from build123d import *

# Parameters (mm, degrees)
F2_R = 10


with BuildPart() as f1:
    # F0 (on Front) → F1 (revolve)
    with BuildSketch(Plane.XZ):
        with BuildLine():
            Line((-119.485281, 0), (-30, 0))
            Line((-30, 0), (-30, 75))
            ThreePointArc((-30, 75), (-33.703899, 80.543277), (-40.242641, 79.242641))
            Line((-40.242641, 79.242641), (-119.485281, 0))
        make_face()
    revolve(axis=Axis((0, 0, 64.130453), (0, 0, 1)))

    # F2 (on Front) → F3 (revolve, cut)
    with BuildSketch(Plane.XZ):
        with Locations((-70, 50)):
            Circle(F2_R)
    revolve(axis=Axis((0, 0, 64.130453), (0, 0, 1)), mode=Mode.SUBTRACT)


solid = f1.part
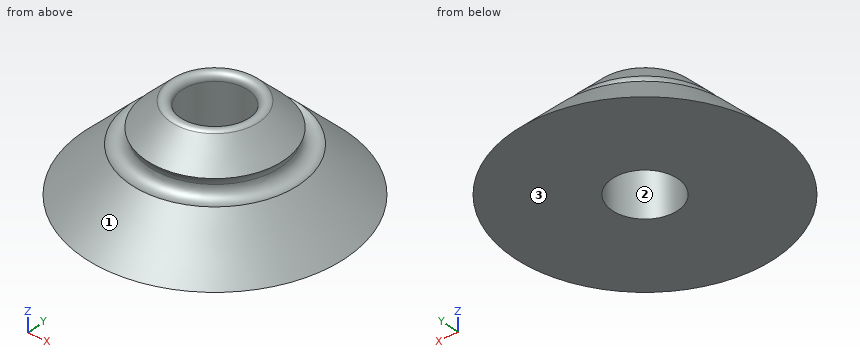
Read the model definition and answer for the solid it produces. Units are mm, in the model's axes. Face numbers are marked on the shaded views. Coordinates: 2 decimals unless noted, no trailing zeros. Loops run counter-clockwise (first coordinate to the right, second up) from the corner with the lowest first, then second, coordinate; pieces in that order, holes last.
Q1. Each of these flat-tipped pins is pushed along its axis until it touches: pin 1 Ø5 at (y, z) = (-65.5, 21) entering from +X; pin 2 Ø1 at (y, z) = (15.5, 29.5) entering from +X; pin 3 Ø5 at (x, z) = (-45, 32) entering from -Y. Where does it stop, or does it pass through?
Q2. The part is cut by section A-A on y = 0. Write down the section's boundary in (x, z).
Q3. The mould has two halves that part along Y. Classify the marked faces 1, 2 and 3: +Y half, -Y half, draft (parallel to the pull), parting line (faces both ways), or undercut.
Q4. The part is cut by section C-C on z = 37. Write down the section's boundary in (x, y), and give its area (3 significant figures).
Q5. Consider probe 1 along Y at (x, z) = (-11.5, 42); probe 2 along X at (y, z) = (0, 16); probe 3 along Y at (x, z) = (0, 35). Determine where each line is inside the solid, lowest interval first.
Results below:
1. pin 1: stops at x = 77.48
1. pin 2: stops at x = 89.16
1. pin 3: stops at y = -78.26
2. outline: (-119.49, 0) - (-30, 0) - (-30, 75) arc R6 ccw to (-40.24, 79.24) - (-62.68, 56.81) arc R10 cw to (-76.81, 42.68) - close; (30, 0) - (119.49, 0) - (76.81, 42.68) arc R10 cw to (62.68, 56.81) - (40.24, 79.24) arc R6 ccw to (30, 75) - close
3. face 1: parting line
3. face 2: undercut
3. face 3: draft
4. outline: circle Ø164.97 at (0, 0); hole circle Ø60 at (0, 0)
4. area: 18,500 mm2
5. probe 1: y = -76.63 to -75.12, -62.96 to -27.71, 27.71 to 62.96, 75.12 to 76.63
5. probe 2: x = -103.49 to -30, 30 to 103.49
5. probe 3: y = -84.49 to -30, 30 to 84.49
